from build123d import *

# Parameters (mm, degrees)
F0_W           = 135
F0_H           = 100
F1_DEPTH       = 10
F4_D           = 6.6
F4_CBORE_D     = 11.25
F4_CBORE_DEPTH = 6
F5_R           = 5
F7_D           = 3.4
F7_CSINK_D     = 6.72
F7_CSINK_ANGLE = 90


with BuildPart() as f1:
    # F0 (on Top) → F1 (new body)
    with BuildSketch(Plane.XY):
        with Locations((67.5, 50)):
            Rectangle(F0_W, F0_H)
    extrude(amount=F1_DEPTH)

    # F4 (through all)
    with Locations(Plane.XY.offset(10)):
        with Locations((12.3223304703, 67.0123483286), (47.6776695297, 67.0123483286), (47.6776695297, 31.6570092693), (12.3223304703, 31.6570092693)):
            CounterBoreHole(F4_D / 2, F4_CBORE_D / 2, F4_CBORE_DEPTH)

    # F5
    f5_edges = [f1.edges().sort_by_distance(p)[0] for p in [
        (0, 100, 5),
        (135, 100, 5),
        (135, 0, 5),
        (0, 0, 5),
    ]]
    fillet(f5_edges, radius=F5_R)

    # F7 (through all)
    with Locations(Plane.XY.offset(10)):
        with Locations((86.5, 20.75), (86.5, 79.25), (125, 79.25), (125, 20.75)):
            CounterSinkHole(F7_D / 2, F7_CSINK_D / 2, counter_sink_angle=F7_CSINK_ANGLE)


solid = f1.part
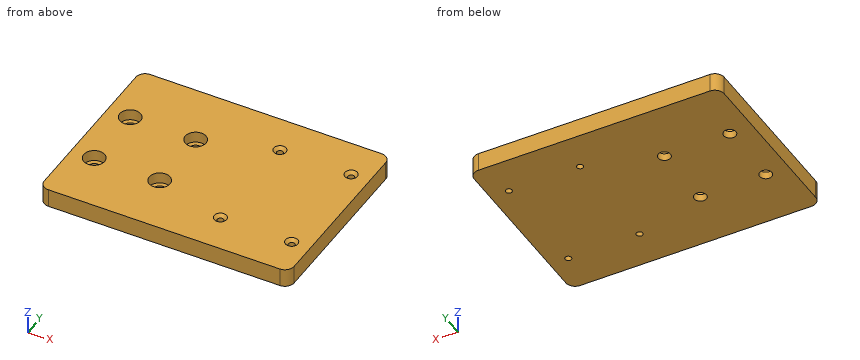
Build history of the part. All positions in model axes, mm. Coordinates: 2 decimals unless noted, no trailing zeros. Write each loop counter-clockwise with the first axis right and the second up, starting at its lowest first coordinate (ties: lowest second). Pieces come first, ordered by that corner, then holes.
(1) Pin check, flat tips, straight feed: pin 1 Ø14.5 at (x, y) = (47.68, 67.01) entering from +Z; pin 2 Ø3.5 at (x, y) = (45, 69) entering from +Z. Stop position of each tip, or through.
(2) Cut at B-B on x = 125. List the corners of the cut face in (y, z).
(3) Cut at A-A on y = 79.25. List the corners of the cut face in (x, z).
(4) Drill centre lines: line 1 (Y direction, x = 86.5, z = 0.75); line 2 (Y direction, x = 85.5, z = 9.75); line 3 (X direction, y = 96.5, z = 6). Where is each one in solid material? Low to high.
Working result:
1. pin 1: stops at z = 10
1. pin 2: stops at z = 4
2. outline: (0, 0) - (19.05, 0) - (19.05, 8.34) - (17.39, 10) - (0, 10) - close; (22.45, 0) - (77.55, 0) - (77.55, 8.34) - (75.89, 10) - (24.11, 10) - (22.45, 8.34) - close; (80.95, 0) - (100, 0) - (100, 10) - (82.61, 10) - (80.95, 8.34) - close
3. outline: (0, 0) - (84.8, 0) - (84.8, 8.34) - (83.14, 10) - (0, 10) - close; (88.2, 0) - (123.3, 0) - (123.3, 8.34) - (121.64, 10) - (89.86, 10) - (88.2, 8.34) - close; (126.7, 0) - (135, 0) - (135, 10) - (128.36, 10) - (126.7, 8.34) - close
4. line 1: y = 0 to 19.05, 22.45 to 77.55, 80.95 to 100
4. line 2: y = 0 to 17.81, 23.69 to 76.31, 82.19 to 100
4. line 3: x = 0.23 to 134.77
